Geometry check sheet. Reference: the model listing, model coordinates, mm. Face numbers are marked on the shaded views. A direction names the side the tool comes from. Coordinates: 2 decimals unless noted, no trailing zeros. Loops run counter-clockwise (first coordinate to the right, second up) from the corner with the lowest first, then second, coordinate; pieces in that order, holes last. Notation, with made-up numbers: (46.25, 73.5) - (99.25, 73.5) arc R9 ccw to (99.25, 85.5) - close; hole circle Ø3 at (6.5, 40). An arc over 180 degrees is marked (long way). Write each question's results on one line, items separated by ' | '. Start each with the question number.
(1) Material ranges on probe 1 along Y at (x, z) = (16.5, -1.5); probe 2 along Y at (x, z) = (-47.5, -2.05); probe 3 along Y at (x, z) = (48.5, -1.1), recorded low to high.
(2) Access from +Z, -Z, +X, -X, +Y, -Y to the whole of each face (thin tool, end or side, straight path). Record for the marked faces 1 and 2.
(3) Go/stop test with flat-tipped pins: pin 1 Ø3.5 at (x, z) = (-31.5, -13) entering from +Y; pin 2 Ø4 at (y, z) = (15, -8.5) entering from +X; pin 3 Ø2 at (x, y) = (9, 19) entering from -Z; pin 4 Ø8 at (x, z) = (-31, -17) entering from +Y. Record where each tip stops, or that it passes through.
(4) Sectioned sample at B-B (y = 28). Enter the section's corners in (x, z), plus the area to 3 significant figures.
(5) Sectioned sample at A-A (x = 26.2). Enter the section's corners in (y, z), plus the area to 3 significant figures.
(6) Sectioned sample at C-C (z = -18.25). Enter the section's corners in (x, y).
(7) Sectioned sample at D-D (x = -20). Enter the section's corners in (y, z).
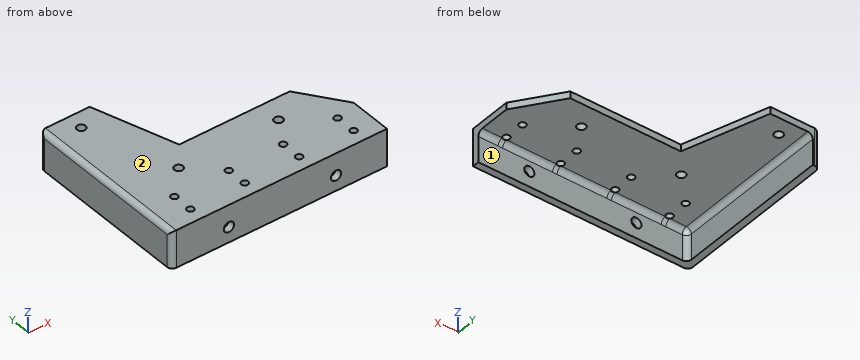
from build123d import *

# Parameters (mm, degrees)
F0_W     = 123
F0_H     = 21
F1_DEPTH = 4
F0_H_2   = 4
F2_DEPTH = 22
F3_D     = 5
F4_D     = 4
F6_D     = 6
F7_R     = 3


with BuildPart() as f1:
    # F0 (on Top) → F1 (new body)
    with BuildSketch(Plane.XY):
        Rectangle(F0_W, F0_H)
        Polygon((-61.5, 10.5), (61.5, 10.5), (43.5, 35.5), (-21.5, 35.5), (-36.5, 83.5), (-61.5, 83.5), align=None)
    extrude(amount=-F1_DEPTH)

    # F0 (on Top) → F2 (join)
    with BuildSketch(Plane.XY):
        Polygon((-61.5, -14.5), (-61.5, -10.5), (-61.5, 10.5), (-61.5, 83.5), (-65.5, 83.5), (-65.5, -14.5), align=None)
        with Locations((0, -12.5)):
            Rectangle(F0_W, F0_H_2)
    extrude(amount=-F2_DEPTH)

    # F3 (through all)
    with Locations(Plane.XY):
        with Locations((-49.3, 73.5), (-32.6, 21.8), (26.2, 21.8)):
            Hole(F3_D / 2)

    # F4 (through all)
    with Locations(Plane.XY):
        with Locations((-47.5, 6), (-47.5, -6), (-15.5, -6), (-15.5, 6), (16.5, -6), (16.5, 6), (48.5, 6), (48.5, -6)):
            Hole(F4_D / 2)

    # F6 (through all)
    with Locations(Plane(origin=(0, -10.5, 0), x_dir=(-1, 0, 0), z_dir=(0, 1, 0))):
        with Locations((-31.5, -13), (31.5, -13)):
            Hole(F6_D / 2)

    # F7
    f7_edges = [f1.edges().sort_by_distance(p)[0] for p in [
        (0, -10.5, -4),
        (-61.5, 36.5, -4),
        (-61.5, -10.5, -13),
        (-65.5, -14.5, -11),
        (-65.5, 34.5, 0),
        (-65.5, 83.5, -11),
    ]]
    fillet(f7_edges, radius=F7_R)


solid = f1.part
Outcome:
1) probe 1: y = -14.5 to -8, -4 to 4, 8 to 35.5 | probe 2: y = -14.5 to -8, -4 to 4, 8 to 71.77, 75.23 to 83.5 | probe 3: y = -14.5 to -8, -4 to 4, 8 to 28.56
2) face 1: -Z, +X, +Y | face 2: +Z, +X, -X, +Y, -Y
3) pin 1: passes through | pin 2: stops at x = -61.46 | pin 3: stops at z = -4 | pin 4: stops at y = -10.5
4) outline: (-65.5, -22) - (-61.5, -22) - (-61.5, -7) arc R3 cw to (-58.5, -4) - (48.9, -4) - (48.9, 0) - (-62.5, 0) arc R3 ccw to (-65.5, -3) - close | area: 530 mm2
5) outline: (-14.5, -22) - (-10.5, -22) - (-10.5, -7) arc R3 cw to (-7.5, -4) - (19.3, -4) - (19.3, 0) - (-14.5, 0) - close; (24.3, -4) - (35.5, -4) - (35.5, 0) - (24.3, 0) - close | area: 254 mm2
6) outline: (-65.5, -11.5) arc R3 ccw to (-62.5, -14.5) - (61.5, -14.5) - (61.5, -10.5) - (-58.5, -10.5) arc R3 cw to (-61.5, -7.5) - (-61.5, 83.5) - (-62.5, 83.5) arc R3 ccw to (-65.5, 80.5) - close
7) outline: (-14.5, -22) - (-10.5, -22) - (-10.5, -7) arc R3 cw to (-7.5, -4) - (35.5, -4) - (35.5, 0) - (-14.5, 0) - close
